from build123d import *

# Parameters (mm, degrees)
SALIENTE_EXTRUIR1_DEPTH = 3
CROQUIS2_R              = 3.7
CROQUIS2_R_2            = 1.5
SALIENTE_EXTRUIR2_DEPTH = 23
CROQUIS3_R              = 1.5
CORTAR_EXTRUIR1_DEPTH   = 3


with BuildPart() as part:
    # Croquis1 → Saliente-Extruir1 (new body)
    with BuildSketch(Plane.XY):
        with BuildLine():
            Line((-194.10496046, 92.470884256), (-194.10496046, 88.470884256))
            Line((-194.10496046, 88.470884256), (-194.10496046, 5.382772077))
            Line((-194.10496046, 5.382772077), (-194.10496046, -1.529115744))
            ThreePointArc((-194.10496046, -1.529115744), (-193.226280804, -3.650436088), (-191.10496046, -4.529115744))
            Line((-191.10496046, -4.529115744), (-165.10496046, -4.529115744))
            ThreePointArc((-165.10496046, -4.529115744), (-162.983640117, -3.650436088), (-162.10496046, -1.529115744))
            Line((-162.10496046, -1.529115744), (-162.10496046, 5.470884256))
            ThreePointArc((-162.10496046, 5.470884256), (-161.226280804, 7.592204599), (-159.10496046, 8.470884256))
            Line((-159.10496046, 8.470884256), (-126.10496046, 8.470884256))
            ThreePointArc((-126.10496046, 8.470884256), (-123.983640117, 7.592204599), (-123.10496046, 5.470884256))
            Line((-123.10496046, 5.470884256), (-123.10496046, -1.529115744))
            ThreePointArc((-123.10496046, -1.529115744), (-122.226280804, -3.650436088), (-120.10496046, -4.529115744))
            Line((-120.10496046, -4.529115744), (-102.10496046, -4.529115744))
            ThreePointArc((-102.10496046, -4.529115744), (-99.983640117, -3.650436088), (-99.10496046, -1.529115744))
            Line((-99.10496046, -1.529115744), (-99.10496046, 22.470884256))
            ThreePointArc((-99.10496046, 22.470884256), (-99.983640117, 24.592204599), (-102.10496046, 25.470884256))
            Line((-102.10496046, 25.470884256), (-111.10496046, 25.470884256))
            ThreePointArc((-111.10496046, 25.470884256), (-113.226280804, 26.349563912), (-114.10496046, 28.470884256))
            Line((-114.10496046, 28.470884256), (-114.10496046, 60.470884256))
            Line((-114.10496046, 60.470884256), (-114.10496046, 83.470884256))
            Line((-114.10496046, 83.470884256), (-102.10496046, 83.470884256))
            ThreePointArc((-102.10496046, 83.470884256), (-99.983640117, 84.349563912), (-99.10496046, 86.470884256))
            Line((-99.10496046, 86.470884256), (-99.10496046, 92.470884256))
            ThreePointArc((-99.10496046, 92.470884256), (-99.983640117, 94.592204599), (-102.10496046, 95.470884256))
            Line((-102.10496046, 95.470884256), (-191.10496046, 95.470884256))
            ThreePointArc((-191.10496046, 95.470884256), (-193.226280804, 94.592204599), (-194.10496046, 92.470884256))
        make_face()
        with BuildLine():
            Line((-181.973694619, 53.715677144), (-191.512513703, 53.715677144))
            ThreePointArc((-191.512513703, 53.715677144), (-171.693012047, 84.571249386), (-135.061551809, 86.307655189))
            Line((-135.061551809, 86.307655189), (-139.830961352, 78.04679554))
            Line((-139.830961352, 78.04679554), (-148.106714986, 63.712769774))
            ThreePointArc((-148.106714986, 63.712769774), (-159.262513703, 63.040994691), (-165.422187349, 53.715677144))
            Line((-165.422187349, 53.715677144), (-181.973694619, 53.715677144))
        make_face(mode=Mode.SUBTRACT)
        with BuildLine():
            Line((-145.508638775, 62.212769774), (-137.23288514, 76.54679554))
            Line((-137.23288514, 76.54679554), (-132.463475598, 84.807655189))
            ThreePointArc((-132.463475598, 84.807655189), (-115.651517015, 52.215677144), (-132.463475598, 19.623699098))
            Line((-132.463475598, 19.623699098), (-137.23288514, 27.884558748))
            Line((-137.23288514, 27.884558748), (-145.508638775, 42.218584514))
            ThreePointArc((-145.508638775, 42.218584514), (-140.512513703, 52.215677144), (-145.508638775, 62.212769774))
        make_face(mode=Mode.SUBTRACT)
        with BuildLine():
            Line((-148.106714986, 40.718584514), (-139.830961352, 26.384558748))
            Line((-139.830961352, 26.384558748), (-135.061551809, 18.123699098))
            ThreePointArc((-135.061551809, 18.123699098), (-171.693012047, 19.860104901), (-191.512513703, 50.715677144))
            Line((-191.512513703, 50.715677144), (-181.973694619, 50.715677144))
            Line((-181.973694619, 50.715677144), (-165.422187349, 50.715677144))
            ThreePointArc((-165.422187349, 50.715677144), (-159.262513703, 41.390359596), (-148.106714986, 40.718584514))
        make_face(mode=Mode.SUBTRACT)
    extrude(amount=SALIENTE_EXTRUIR1_DEPTH)

    # Croquis2 → Saliente-Extruir2 (add)
    with BuildSketch(Plane(origin=(0, 0, 0), x_dir=(-1, 0, 0), z_dir=(0, 0, -1))):
        with Locations((189.10496046, 90.470884256)):
            Circle(CROQUIS2_R)
        with Locations((189.10496046, 90.470884256)):
            Circle(CROQUIS2_R_2, mode=Mode.SUBTRACT)
        with Locations((104.10496046, 90.470884256)):
            Circle(CROQUIS2_R)
        with Locations((104.10496046, 90.470884256)):
            Circle(CROQUIS2_R_2, mode=Mode.SUBTRACT)
        with Locations((104.10496046, 0.470884256)):
            Circle(CROQUIS2_R)
        with Locations((104.10496046, 0.470884256)):
            Circle(CROQUIS2_R_2, mode=Mode.SUBTRACT)
        with Locations((189.10496046, 0.470884256)):
            Circle(CROQUIS2_R)
        with Locations((189.10496046, 0.470884256)):
            Circle(CROQUIS2_R_2, mode=Mode.SUBTRACT)
    extrude(amount=SALIENTE_EXTRUIR2_DEPTH)

    # Croquis3 → Cortar-Extruir1 (cut)
    with BuildSketch(Plane.XY.offset(3)):
        with Locations((-117.012513703, 16.215677144)):
            Circle(CROQUIS3_R)
        with Locations((-189.012513703, 16.215677144)):
            Circle(CROQUIS3_R)
        with Locations((-117.012513703, 88.215677144)):
            Circle(CROQUIS3_R)
    extrude(amount=-CORTAR_EXTRUIR1_DEPTH, mode=Mode.SUBTRACT)


solid = part.part
The listing builds one solid part. Answer for the finished solid, in the listing's coordinates (mm). A direction names the side the tool comes from. Round coordinates to 2 decimals unless told otherwise and drop trailing zeros. Write each loop counter-clockwise with the first axis right and the second up, starting at its lowest first coordinate (ties: lowest second). Pieces come first, ordered by that corner, then holes. Notation, with made-up numbers: (17, 7.25) - (58, 7.25) arc R18 cw to (58, 37.25) - close; hole circle Ø10 at (25, 86.25). An arc over 180 degrees is marked (long way). Use a Markdown table: item, result. Add a question column.
1. A tool of negligible diameter and unlimited length cuts with its end or side. For faces 1 (the face through (-107.634, 91.582, -11.339)), 2 (the face through (-178, 53.716, 1)), 3 (the face through (-122.249, -3.627, 1.479)), 4 (the face through (-147, 46, 3)), from which of +Z, -Z, +X, -X, +Y, -Y can it reach the whole face along a straight path? Write none if from no direction.
2. The part is cut by section C-C (x = -112.5). Write down the section's boundary in (y, z).
3. The part is cut by section A-A (z = -12.25). Write down the section's boundary in (x, y).
4. For a pull along X with two mould halves and no side action, classify faces 5 (the face through (-193.2, 94.62, 1.48)), 6 (the face through (-159.12, 63.12, 1.48)), 7 (the face through (-106, 1, -23)) as +X half, -X half, draft (parallel to the pull), parting line (faces both ways), or undercut.
5. The part is cut by section D-D (x = -177). Write down the section's boundary in (y, z), and give its area (3 significant figures).
6. The part is cut by section B-B (y = 60). Write down the section's boundary in (x, z), and give its area (3 significant figures).
7. Flat-ended cylindrical pins translate along their axes: P1, Ø1.5, axis at x = -144.5, z = 1.5, coming from the -Y side; P2, Ø0.9, axis at x = -105, y = 0.5, coming from the -Z side. Find the tip coordinate at first contact, or state that the pin passes through.
8. Consider line 1 (Y direction, x = -139, z = 1.5); line 2 (Y direction, x = -106, z = 1.75); line 3 (Y direction, x = -105, z = -17.75). Determine where each line is inside the solid, lowest interval first.
Reported:
| question | item | result |
|---|---|---|
| 1 | face 1 | -Z |
| 1 | face 2 | +Z, -Z |
| 1 | face 3 | +Z, -Z, -Y |
| 1 | face 4 | +Z, +X, -X, +Y, -Y |
| 2 | outline | (-4.53, 0) - (25.81, 0) - (25.81, 3) - (-4.53, 3) - close; (83.47, 0) - (95.47, 0) - (95.47, 3) - (83.47, 3) - close |
| 3 | outline | circle Ø7.4 at (-189.1, 0.47); circle Ø7.4 at (-189.1, 90.47); circle Ø7.4 at (-104.1, 0.47); circle Ø7.4 at (-104.1, 90.47); hole circle Ø3 at (-189.1, 0.47); hole circle Ø3 at (-189.1, 90.47); hole circle Ø3 at (-104.1, 0.47); hole circle Ø3 at (-104.1, 90.47) |
| 4 | face 5 | -X half |
| 4 | face 6 | undercut |
| 4 | face 7 | draft |
| 5 | outline | (-4.53, 0) - (23.52, 0) - (23.52, 3) - (-4.53, 3) - close; (50.72, 0) - (53.72, 0) - (53.72, 3) - (50.72, 3) - close; (80.91, 0) - (95.47, 0) - (95.47, 3) - (80.91, 3) - close |
| 5 | area | 137 mm^2 |
| 6 | outline | (-194.1, 0) - (-190.4, 0) - (-190.4, 3) - (-194.1, 3) - close; (-162.79, 0) - (-143.23, 0) - (-143.23, 3) - (-162.79, 3) - close; (-116.42, 0) - (-114.1, 0) - (-114.1, 3) - (-116.42, 3) - close |
| 6 | area | 76.7 mm^2 |
| 7 | P1 | y = 8.47 |
| 7 | P2 | z = 0 |
| 8 | line 1 | 8.47 to 16.57, 24.95 to 30.95, 73.49 to 79.49, 87.86 to 95.47 |
| 8 | line 2 | -4.53 to 25.47, 83.47 to 95.47 |
| 8 | line 3 | -3.12 to -0.73, 1.67 to 4.06, 86.88 to 89.27, 91.67 to 94.06 |
